Work out the finished part from the listing and answer in its coordinate system (mm). A direction names the side the tool comes from. Coordinates: 2 decimals unless noted, no trailing zeros. Write each loop counter-clockwise with the first axis right and the second up, starting at its lowest first coordinate (ties: lowest second). Pieces come first, ordered by that corner, then holes. Notation, with made-up numbers: (46.5, 59) - (86.5, 59) arc R10 cw to (86.5, 71) - close; hole circle Ø8 at (49, 30.5). An arc over 180 degrees is marked (long way). Answer as a JSON object with one key per item and string values. Group by question number.
Autodesk Inventor part; units mm, degrees
ref_plane "YZ Plane" through (0, 0, 0) normal (1, 0, 0) x (0, 1, 0)
ref_plane "XZ Plane" through (0, 0, 0) normal (0, 1, 0) x (-1, 0, 0)
ref_plane "XY Plane" through (0, 0, 0) normal (0, 0, 1) x (1, 0, 0)
sketch "Sketch1" plane through (0, 0, 0) normal (0, 0, 1) x (1, 0, 0)
  line L0 (-78.24, 3.5741) -> (4.16, 3.5741)
  line L1 (4.16, 3.5741) -> (4.16, -28.8259)
  line L2 (4.16, -28.8259) -> (-78.24, -28.8259)
  line L3 (-78.24, -28.8259) -> (-78.24, 3.5741)
  line L4 (-77.04, 2.3741) -> (2.96, 2.3741)
  line L5 (2.96, 2.3741) -> (2.96, -27.6259)
  line L6 (2.96, -27.6259) -> (-77.04, -27.6259)
  line L7 (-77.04, -27.6259) -> (-77.04, 2.3741)
  point P0 (0, 0)
  dimension "d0" = 32.4
  dimension "d1" = 82.4
  dimension "d2" = 1.2
  dimension "d3" = 1.2
  dimension "d4" = 1.2
  dimension "d5" = 1.2
extrude "Extrusion1" add sketch "Sketch1" along normal blind 25
sketch "Sketch2" plane through (0, 0, 25) normal (0, 0, 1) x (1, 0, 0)
  line L0 (-78.24, 3.5741) -> (4.16, 3.5741)
  line L1 (4.16, 3.5741) -> (4.16, -28.8259)
  line L2 (4.16, -28.8259) -> (-78.24, -28.8259)
  line L3 (-78.24, -28.8259) -> (-78.24, 3.5741)
  point P0 (0, 0)
extrude "Extrusion2" add sketch "Sketch2" along normal blind 1.2
sketch "Sketch3" plane through (-78.24, -28.8259, 0) normal (-1, 0, 0) x (0, 0, 1)
  line L0 (25, 1.2) -> (25, 31.2)
  line L1 (25, 12.45) -> (22, 12.45)
  line L2 (22, 12.45) -> (22, 19.95)
  line L3 (22, 19.95) -> (25, 19.95)
  line L4 (25, 19.95) -> (25, 12.45)
  line L5 (0, 1.2) -> (25, 1.2)
  line L6 (0, 31.2) -> (25, 31.2)
  point P0 (0, 28.8259)
  dimension "d10" = 7.5
  dimension "d11" = 3
  dimension "d12" = 11.25
  dimension "d13" = 11.25
extrude "Extrusion3" cut sketch "Sketch3" against normal blind 1.2
sketch "Sketch4" plane through (0, 0, 25) normal (0, 0, -1) x (-1, 0, 0)
  point P0 (0, 0)
sketch "Sketch5" plane through (0, 0, 25) normal (0, 0, -1) x (-1, 0, 0)
  line L0 (18.04, -7.6259) -> (19.04, -7.6259)
  line L1 (19.04, -7.6259) -> (19.04, -17.6259)
  line L2 (19.04, -17.6259) -> (18.04, -17.6259)
  line L3 (18.04, -17.6259) -> (18.04, -7.6259)
  line L4 (-2.96, 2.3741) -> (77.04, 2.3741)
  line L5 (77.04, -27.6259) -> (-2.96, -27.6259)
  line L6 (77.04, 2.3741) -> (77.04, -27.6259)
  point P0 (0, 0)
  dimension "d16" = 1
  dimension "d17" = 10
  dimension "d18" = 10
  dimension "d19" = 10
  dimension "d20" = 58
extrude "Extrusion4" add sketch "Sketch5" along normal blind 1.5
chamfer "Chamfer1" distance 1.5 angle 45 2 edges at (-18.54, -17.6259, 23.5) (-18.54, -7.6259, 23.5)
chamfer "Chamfer2" distance 1.5 angle 45 1 edges at (-18.04, -12.6259, 25)
sketch "Sketch6" plane through (-78.24, -28.8259, 0) normal (0, -1, 0) x (1, 0, 0)
  circle A0 centre (3.7, 12.5) radius 2.5
  line L0 (1.2, 0) -> (1.2, 25)
  point P0 (78.24, 0)
  dimension "d29" = 5
  dimension "d30" = 2.5
extrude "Extrusion5" cut sketch "Sketch6" against normal blind 40
sketch "Sketch7" plane through (4.16, -28.8259, 0) normal (1, 0, 0) x (0, 0, -1)
  line L0 (0, 31.2) -> (-25, 31.2)
  line L1 (0, 32.4) -> (0, 0)
  circle A0 centre (-8, 26.2) radius 1.5
  circle A1 centre (-8, 21.2) radius 1.5
  circle A2 centre (-8, 16.2) radius 1.5
  circle A3 centre (-8, 11.2) radius 1.5
  circle A4 centre (-8, 6.2) radius 1.5
  line L2 (0, 1.2) -> (-25, 1.2)
  point P0 (0, 28.8259)
  point P1 (-8, 31.2)
  dimension "d33" = 8
  dimension "d34" = 3
  dimension "d35" = 3
  dimension "d36" = 3
  dimension "d37" = 3
  dimension "d38" = 3
  dimension "d39" = 5
  dimension "d40" = 5
  dimension "d41" = 5
  dimension "d42" = 5
  dimension "d43" = 5
  dimension "d44" = 5
extrude "Extrusion6" cut sketch "Sketch7" against normal blind 3
properties part number "Case Botom"
Q1. Section B-B on x = -74.54 is taken. Determine the outline of the cut face in (y, z), plus the area to 3 significant figures.
Q2. Consider L1, parallel to Y at x = 3.8, z = 8; L2, parallel to Y at x = -68, z = 21.75; L3, parallel to X at y = -27, z = 6.25. Determine where each line is inside the solid, lowest interval first. Write a range as from..to.
Q3. Section C-C on z = 2 is taken. Determine the outline of the cut face in (x, y).
Q4. Flat-ended cylindrical pins translate along their axes: pin 1 Ø4.5 at (x, z) = (-74.54, 12.5) entering from -Y (3 decimals); pin 2 Ø0.5 at (x, y) = (-19, -13.5) entering from -Z; pin 3 Ø12 at (x, y) = (-11, -10) entering from -Z; pin 4 Ø1.5 at (x, y) = (-54, -19.5) entering from -Z. Find the tip coordinate at first contact, or state that the pin passes through.
Q5. Section D-D on x = -15.5 is taken. Determine the outline of the cut face in (y, z).
Q6. For a pull along X with two mould halves and no side action, classify faces 4 (the face through (4.16, -12, 13)), 5 (the face through (3.6, -12.6, 9.5)), 6 (the face through (-73.39, -28.23, 10.28)) as +X half, -X half, draft (parallel to the pull), parting line (faces both ways), or undercut.
Q7. Section A-A on z = 8 is taken. Determine the outline of the cut face in (x, y).
Q8. A tool of negligible diameter and unlimited length cuts with its end or side. For faces 1 (the face through (3.568, -21.612, 9.106)), 2 (the face through (-18.05, -17.032, 24.406)), 3 (the face through (-38, -12, 26.2)), from which of +Z, -Z, +X, -X, +Y, -Y can it reach the whole face along a straight path? Write none if from no direction.
Numbers:
{
 "1": {"outline": "(-28.83, 0) - (-27.63, 0) - (-27.63, 10) - (-28.83, 10) - close; (-28.83, 15) - (-27.63, 15) - (-27.63, 25) - (2.37, 25) - (2.37, 15) - (3.57, 15) - (3.57, 26.2) - (-28.83, 26.2) - close; (2.37, 0) - (3.57, 0) - (3.57, 10) - (2.37, 10) - close", "area": "86.9 mm²"},
 "2": {"L1": "y = -28.83..-24.13, -21.13..-19.13, -16.13..-14.13, -11.13..-9.13, -6.13..-4.13, -1.13..3.57", "L2": "y = -28.83..-27.63, 2.37..3.57", "L3": "x = -78.24..-77.04, 2.96..4.16"},
 "3": {"outline": "(-78.24, -28.83) - (4.16, -28.83) - (4.16, 3.57) - (-78.24, 3.57) - close; hole (-77.04, -27.63) - (2.96, -27.63) - (2.96, 2.37) - (-77.04, 2.37) - close"},
 "4": {"pin 1": "passes through", "pin 2": "stops at z = 23.5", "pin 3": "stops at z = 24.54", "pin 4": "stops at z = 25"},
 "5": {"outline": "(-28.83, 0) - (-27.63, 0) - (-27.63, 25) - (2.37, 25) - (2.37, 0) - (3.57, 0) - (3.57, 26.2) - (-28.83, 26.2) - close"},
 "6": {"face 4": "+X half", "face 5": "draft", "face 6": "undercut"},
 "7": {"outline": "(-78.24, -28.83) - (4.16, -28.83) - (4.16, -24.13) - (2.96, -24.13) - (2.96, -27.63) - (-77.04, -27.63) - (-77.04, 2.37) - (2.96, 2.37) - (2.96, -1.13) - (4.16, -1.13) - (4.16, 3.57) - (-78.24, 3.57) - close; (2.96, -21.13) - (4.16, -21.13) - (4.16, -19.13) - (2.96, -19.13) - close; (2.96, -16.13) - (4.16, -16.13) - (4.16, -14.13) - (2.96, -14.13) - close; (2.96, -11.13) - (4.16, -11.13) - (4.16, -9.13) - (2.96, -9.13) - close; (2.96, -6.13) - (4.16, -6.13) - (4.16, -4.13) - (2.96, -4.13) - close"},
 "8": {"face 1": "+X", "face 2": "-Z", "face 3": "+Z, +X, -X, +Y, -Y"}
}
